Verification items for the finished model (mm, model axes). Face numbers are marked on the shaded views. A direction names the side the tool comes from. Coordinates: 2 decimals unless noted, no trailing zeros. Order: outer loops, then holes, each group sorted by start corner. A loop starts at its lowest first (then second) coordinate and runs counter-clockwise, first axis right, second up. Notation, with made-up numbers: M 41.5,-19.5 L 62.5,-19.5 A15 cw 62.5,0.5 Z; hole C 84,-13 d8. An arc over 180 degrees is marked long. Return JSON: item names as keys, results as strings.
```python
from build123d import *

# Parameters (mm, degrees)
SKETCH_1_W             = 29
SKETCH_1_H             = 15
EXTRUDE_1_DEPTH        = 2
SKETCH_2_W             = 8.2
SKETCH_2_H             = 20.4
SKETCH_2_R             = 2.15
EXTRUDE_2_DEPTH        = 2.5
EXTRUDE_3_DEPTH        = 2
FILLET_1_R             = 1
FILLET_1_OF_MIRROR_2_R = 1


with BuildPart() as part:
    # 草图1 → 凸台-拉伸1 (new body)
    with BuildSketch(Plane.XY):
        with Locations((-14.5, 7.5)):
            Rectangle(SKETCH_1_W, SKETCH_1_H)
    extrude_1 = extrude(amount=EXTRUDE_1_DEPTH)

    # 草图2 → 凸台-拉伸2 (add)
    with BuildSketch(Plane(origin=(0, 15, 0), x_dir=(1, 0, 0), z_dir=(0, 1, 0))):
        with Locations((-24.9, 10.2)):
            Rectangle(SKETCH_2_W, SKETCH_2_H)
        with Locations((-24.3, 5.5)):
            Circle(SKETCH_2_R, mode=Mode.SUBTRACT)
        with Locations((-24.3, 15.4)):
            Circle(SKETCH_2_R, mode=Mode.SUBTRACT)
    extrude_2 = extrude(amount=-EXTRUDE_2_DEPTH)

    # 草图3 → 凸台-拉伸3 (add)
    with BuildSketch(Plane.ZY.offset(29)):
        Polygon((-20.4, 12.5), (0, 0), (0, 12.5), align=None)
        Polygon((2, 0), (2, 15), (-20.4, 15), (-20.4, 12.5), (0, 12.5), (0, 0), align=None)
    extrude_3 = extrude(amount=EXTRUDE_3_DEPTH)

    # 圆角1
    fillet_1_edges = [part.edges().sort_by_distance(p)[0] for p in [
        (-29, 6.25, 0),
        (-20.8, 13.75, 0),
        (-20.8, 13.75, -20.4),
        (-24.9, 12.5, 0),
        (-29, 12.5, -10.2),
        (-31, 13.75, -20.4),
    ]]
    fillet(fillet_1_edges, radius=FILLET_1_R)

    # 镜向2: 凸台-拉伸1, 凸台-拉伸2, 凸台-拉伸3 across plane
    add(extrude_1.mirror(Plane(origin=(0, 0, 2), x_dir=(0, 0, 1), z_dir=(-1, 0, 0))))
    add(extrude_2.mirror(Plane(origin=(0, 0, 2), x_dir=(0, 0, 1), z_dir=(-1, 0, 0))))
    add(extrude_3.mirror(Plane(origin=(0, 0, 2), x_dir=(0, 0, 1), z_dir=(-1, 0, 0))))

    # 圆角1 of 镜向2
    fillet_1_of_mirror_2_edges = [part.edges().sort_by_distance(p)[0] for p in [
        (29, 6.25, 0),
        (20.8, 13.75, 0),
        (20.8, 13.75, -20.4),
        (24.9, 12.5, 0),
        (29, 12.5, -10.2),
        (31, 13.75, -20.4),
    ]]
    fillet(fillet_1_of_mirror_2_edges, radius=FILLET_1_OF_MIRROR_2_R)


solid = part.part
```
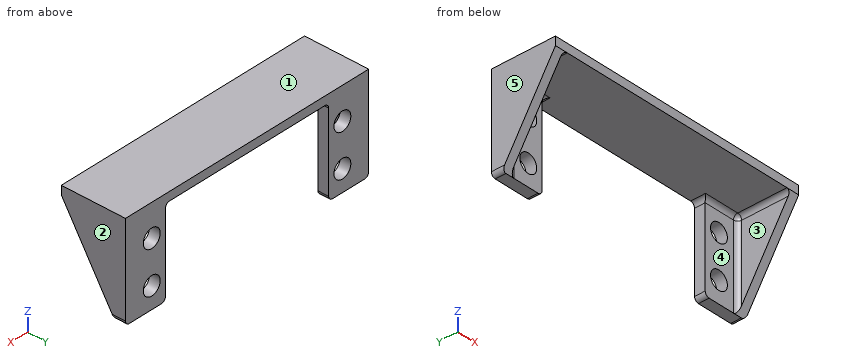
Q1. Material ranges on line 1 along Z through (x, y) = (-24.3, 13); line 2 along X through (y, z) = (1.75, -1.5); line 3 along Z through (x, y) = (15.5, 7), recorded low to high.
Values:
{"line 1": "-20.4 to -17.55, -13.25 to -7.65, -3.35 to 2", "line 2": "-31 to -29, 29 to 31", "line 3": "0 to 2"}
Q2. Cross-section at C-C, the plane y = 1.25. Record the boundary of the cut face in (x, z), and give its area (3 significant figures).
Values:
{"outline": "M -31,-2.04 L -29,-2.04 L -29,-1 A1 cw -28,0 L 28,0 A1 cw 29,-1 L 29,-2.04 L 31,-2.04 L 31,2 L -31,2 Z", "area": "133 mm^2"}
Q3. Draft check along X on the marked faces 1, 2 and 3. Enter one of: pulls with the +X half, pulls with the -X half, needs draft (parallel to the pull), parting line crosses it, or undercut.
Values:
{"face 1": "needs draft", "face 2": "pulls with the +X half", "face 3": "undercut"}
Q4. Tool access check on the marked faces 4 and 5. Record the directions out of +Z, -Z, +X, -X, +Y, -Y that give a thin tool (end or side, any length) a straight path to the whole face; none if there is none.
Values:
{"face 4": "-Z, -Y", "face 5": "+Z, -Z, -X, +Y, -Y"}
Q5. Cross-section at B-B, the plane z = -5.5. Record the boundary of the cut face in (x, y), and give its area (3 significant figures).
Values:
{"outline": "M -31,3.37 L -29,3.37 L -29,11.5 A1 cw -28,12.5 L -26.45,12.5 L -26.45,15 L -31,15 Z; M -22.15,12.5 L -20.8,12.5 L -20.8,15 L -22.15,15 Z; M 20.8,12.5 L 22.15,12.5 L 22.15,15 L 20.8,15 Z; M 26.45,12.5 L 28,12.5 A1 cw 29,11.5 L 29,3.37 L 31,3.37 L 31,15 L 26.45,15 Z", "area": "66.4 mm^2"}
Q6. Go/stop test with flat-tipped pins: pin 1 (2 mm diameter, centred on x = -17, y = 7, fed in from -Z); pin 2 (5.5 mm diameter, centred on x = 24.3, z = -5.5, fed in from +Y); pin 3 (2 mm diameter, centred on x = -23.5, z = -9.5, fed in from -Y); pin 4 (3.5 mm diameter, centred on x = 24.3, z = -15.4, fed in from +Y). Record where each tip stops, or that it passes through.
Values:
{"pin 1": "z = 0", "pin 2": "y = 15", "pin 3": "y = 12.5", "pin 4": "through"}
Q7. Cross-section at A-A, the plane x = 24.3. Record the boundary of the cut face in (y, z), and give its area (3 significant figures).
Values:
{"outline": "M 0,0 L 11.5,0 A1 cw 12.5,-1 L 12.5,-3.35 L 15,-3.35 L 15,2 L 0,2 Z; M 12.5,-20.4 L 15,-20.4 L 15,-17.55 L 12.5,-17.55 Z; M 12.5,-13.25 L 15,-13.25 L 15,-7.65 L 12.5,-7.65 Z", "area": "59.7 mm^2"}
Q8. Cross-section at D-D, the plane z = -15.4. Record the boundary of the cut face in (x, y), and give its area (3 significant figures).
Values:
{"outline": "M -31,9.44 L -29,9.44 L -29,11.5 A1 cw -28,12.5 L -26.45,12.5 L -26.45,15 L -31,15 Z; M -22.15,12.5 L -20.8,12.5 L -20.8,15 L -22.15,15 Z; M 20.8,12.5 L 22.15,12.5 L 22.15,15 L 20.8,15 Z; M 26.45,12.5 L 28,12.5 A1 cw 29,11.5 L 29,9.44 L 31,9.44 L 31,15 L 26.45,15 Z", "area": "42.2 mm^2"}
